Source: CAD feature listing. Evaluate the final solid. Frame: model axes, mm. A direction names the side the tool comes from. Coordinates: 2 decimals unless noted, no trailing zeros. Write each loop counter-clockwise with the first axis right and the second up, starting at its lowest first coordinate (ties: lowest second). Pieces come first, ordered by that corner, then holes. Notation, with made-up numbers: (-29, 36.25) - (-17, 36.25) arc R28 cw to (-17, 62.25) - close; hole circle Ø6 at (0, 31.5). An arc over 180 degrees is marked (long way). One line per item, written item: value.
from build123d import *

# Parameters (mm, degrees)
ESQUISSE1_W                 = 50.8
ESQUISSE1_H                 = 50.8
BOSS_EXTRU_1_DEPTH          = 50.8
TROU_TARAUD_M61_D           = 5
TROU_TARAUD_M61_CSINK_D     = 6.05
TROU_TARAUD_M61_CSINK_ANGLE = 90
ENL_V_MAT_EXTRU_2_REACH     = 89.988


with BuildPart() as part:
    # Esquisse1 → Boss.-Extru.1 (new body)
    with BuildSketch(Plane.XY):
        with Locations((-25.4, 25.4)):
            Rectangle(ESQUISSE1_W, ESQUISSE1_H)
    extrude(amount=BOSS_EXTRU_1_DEPTH)

    # Trou taraudé M61 (through all)
    with Locations(Plane(origin=(0, 50.8, 0), x_dir=(1, 0, 0), z_dir=(0, 1, 0))):
        with Locations((-42.238223885, -7.663368272), (-7.652573676, -7.663368272), (-7.652573676, -43.63244449), (-42.238223885, -43.63244449)):
            CounterSinkHole(TROU_TARAUD_M61_D / 2, TROU_TARAUD_M61_CSINK_D / 2, counter_sink_angle=TROU_TARAUD_M61_CSINK_ANGLE)

    # Esquisse4 → Enlèv. mat.-Extru.2 (cut, up to next)
    with BuildSketch(Plane(origin=(0, 0, 0), x_dir=(0, 0, -1), z_dir=(1, 0, 0)), mode=Mode.PRIVATE) as enl_v_mat_extru_2_sk1:
        with BuildLine():
            Line((-46.721032859, 46.906628003), (-39.78616404, 46.906628003))
            ThreePointArc((-39.78616404, 46.906628003), (-38.679536037, 45.8), (-39.78616404, 44.693371997))
            Line((-39.78616404, 44.693371997), (-46.721032859, 44.693371997))
            ThreePointArc((-46.721032859, 44.693371997), (-47.827660862, 45.8), (-46.721032859, 46.906628003))
        make_face()
    enl_v_mat_extru_2_tool1 = extrude(enl_v_mat_extru_2_sk1.sketch, amount=-ENL_V_MAT_EXTRU_2_REACH, mode=Mode.PRIVATE) & part.part
    add(enl_v_mat_extru_2_tool1.solids().sort_by_distance((0, 45.8, 43.253598))[0], mode=Mode.SUBTRACT)


solid = part.part
1) Material intervals for line 1 (Y direction, x = -30, z = 41.5); line 2 (Z direction, x = -42, y = 28.5); line 3 (Z direction, x = -27.5, y = 46), sorted ascending.
Values found:
line 1: 0 to 44.69, 46.91 to 50.8
line 2: 0 to 5.17, 10.15 to 41.14, 46.12 to 50.8
line 3: 0 to 38.7, 47.81 to 50.8
2) Draft query along Y for faces 3 (the flat face through (-50.8, 25, 25)), 4 (the flat face through (-26, 50.8, 25)), 5 (the cylindrical face through (-25.04, 45.82, 38.68)), 6 (the flat face through (-26, 0, 25)). Return one class per face: released by +Y, released by -Y, zero draft, split by the parting line, or undercut.
Values found:
face 3: zero draft
face 4: released by +Y
face 5: undercut
face 6: released by -Y
3) Section query B-B on y = 33. Output: boundary loops of the cut face in (x, z).
Values found:
outline: (-50.8, 0) - (0, 0) - (0, 50.8) - (-50.8, 50.8) - close; hole circle Ø5 at (-42.24, 7.66); hole circle Ø5 at (-42.24, 43.63); hole circle Ø5 at (-7.65, 7.66); hole circle Ø5 at (-7.65, 43.63)
4) Contact query for a flat-ended pin moving along its axis: P1, Ø4.5, axis at x = -7.65, z = 43.63, coming from the +Y side. Output: stop coordinate, or through.
Values found:
P1: through
5) Reachability of faces 1 (the cylindrical face through (-7.111, 48.567, 46.073)), 2 (the flat face through (-25, 46.907, 43)) from +Z, -Z, +X, -X, +Y, -Y: full face, straight path, thin tool, end or side. Return the list, or none.
Values found:
face 1: +Y, -Y
face 2: +X, -X
6) Section query C-C on z = 44.5. State how many separate pieces and enclosed holes the cut face has, then the cut area to 3 significant figures.
Values found:
separate pieces: 6
enclosed holes: 0
area: 2,010 mm2
7) Section query A-A on y = 45.8. Output: boundary loops of the cut face in (x, z).
Values found:
outline: (-50.8, 0) - (0, 0) - (0, 38.68) - (-50.8, 38.68) - close; (-50.8, 47.83) - (0, 47.83) - (0, 50.8) - (-50.8, 50.8) - close; hole circle Ø5 at (-42.24, 7.66); hole circle Ø5 at (-7.65, 7.66)
